```python
from build123d import *

# Parameters (mm, degrees)
SKETCH_W        = 120
SKETCH_H        = 33
PAD_DEPTH       = 3
SKETCH195_R     = 4
SKETCH195_R_2   = 5
POCKET_DEPTH    = 5
SKETCH196_R     = 1.65
POCKET137_DEPTH = 5
FILLET_R        = 6


with BuildPart() as part:
    # Sketch → Pad (new body)
    with BuildSketch(Plane.XY):
        with Locations((60, -56.515431)):
            Rectangle(SKETCH_W, SKETCH_H)
    extrude(amount=PAD_DEPTH)

    # Sketch195 (on Face6 of Pad) → Pocket (cut)
    with BuildSketch(Plane.XY.offset(3)):
        with Locations((25.000934, -56.019999)):
            Circle(SKETCH195_R)
        with Locations((45.000934, -56.019999)):
            Circle(SKETCH195_R)
        with Locations((70.000934, -56.019999)):
            Circle(SKETCH195_R_2)
        with Locations((95.000934, -56.019999)):
            Circle(SKETCH195_R)
    extrude(amount=-POCKET_DEPTH, mode=Mode.SUBTRACT)

    # Sketch196 (on Face5 of Pocket) → Pocket137 (cut)
    with BuildSketch(Plane.XY.offset(3)):
        with Locations((7.125, -44.415438)):
            Circle(SKETCH196_R)
        with Locations((112.875, -68.713068)):
            Circle(SKETCH196_R)
        with Locations((112.875, -44.415438)):
            Circle(SKETCH196_R)
        with Locations((7.125, -68.713068)):
            Circle(SKETCH196_R)
    extrude(amount=-POCKET137_DEPTH, mode=Mode.SUBTRACT)

    # Fillet
    fillet_edges = [part.edges().sort_by_distance(p)[0] for p in [
        (0, -73.015431, 1.5),
        (0, -40.015431, 1.5),
        (120, -73.015431, 1.5),
        (120, -40.015431, 1.5),
    ]]
    fillet(fillet_edges, radius=FILLET_R)


solid = part.part
```
Verification items for the finished model (mm, model axes). Coordinates: 2 decimals unless noted, no trailing zeros. Loops run counter-clockwise (first coordinate to the right, second up) from the corner with the lowest first, then second, coordinate; pieces in that order, holes last. Notation, with made-up numbers: (28.25, 66.25) - (42.25, 66.25) arc R38 ccw to (42.25, 104.25) - close; hole circle Ø6 at (32.25, -32). An arc over 180 degrees is marked (long way). Return JSON: item names as keys, results as strings.
1. Thickness scan on L1, parallel to Y at x = 45, z = 2.6; L2, parallel to X at y = -57, z = 0.4; L3, parallel to Y at x = 112, z = 2.8. Record the ranges inside material, lowest first.
Established:
{"L1": "y = -73.02 to -60.02, -52.02 to -40.02", "L2": "x = 0 to 21.12, 28.88 to 41.12, 48.88 to 65.1, 74.9 to 91.12, 98.88 to 120", "L3": "y = -73.02 to -70.11, -67.31 to -45.81, -43.02 to -40.02"}
2. Mould release check, pull along X, two halves, no side actions. Record for faces 1 (the cylindrical face through (24.48, -52.054, 1.521)), 2 (the cylindrical face through (1.7, -71.2, 1.5)), 3 (the flat face through (59, -56, 3)): +X half, -X half, draft (parallel to the pull), parting line (faces both ways), or undercut.
Established:
{"face 1": "undercut", "face 2": "-X half", "face 3": "draft"}
3. Section check A-A, the plane x = 95. Record the boundary of the cut face in (y, z), then the cut area to 3 significant figures.
Established:
{"outline": "(-73.02, 0) - (-60.02, 0) - (-60.02, 3) - (-73.02, 3) - close; (-52.02, 0) - (-40.02, 0) - (-40.02, 3) - (-52.02, 3) - close", "area": "75.0 mm2"}
4. Section check B-B, the plane z = 0.6. Count the separate pieces of the cut face and the enclosed holes in it, then the cut area to 3 significant figures.
Established:
{"separate pieces": "1", "enclosed holes": "8", "area": "3,670 mm2"}
5. Go/stop test with a flat-tipped pin: pin 1 (5 mm diameter, centred on x = 25, y = -56.02, fed in from +Z). Record where the tip stops, or that it passes through.
Established:
{"pin 1": "passes through"}
